```python
from build123d import *

# Parameters (mm, degrees)
F0_R      = 53.5
F0_R_2    = 10.9127793542
F1_DEPTH  = 100
F2_R      = 10.9127793542
F3_DEPTH  = 76
F5_R      = 23.9808815671
F5_R_2    = 10.9127793542
F6_DEPTH  = 50
F7_R      = 41.5
F7_R_2    = 23.9808815671
F7_R_3    = 10.9127793542
F8_DEPTH  = 11
F9_R      = 39
F9_R_2    = 10.9127793542
F10_DEPTH = 3
F11_R     = 41.5
F11_R_2   = 39
F11_R_3   = 10.9127793542
F12_DEPTH = 11
F13_R     = 5
F14_DEPTH = 125


# Not quite as in the source:
# - a feature names something its author has since deleted; it is built from what else it names


with BuildPart() as f1:
    # F0 (on Top) → F1 (new body)
    with BuildSketch(Plane.XY):
        Circle(F0_R)
        Circle(F0_R_2, mode=Mode.SUBTRACT)
    extrude(amount=F1_DEPTH)


with BuildPart() as f3:
    # F2 (on face) → F3 (new body)
    with BuildSketch(Plane.XY.offset(100)):
        with BuildLine():
            ThreePointArc((53.5, 0), (49.381382201, 20.5846810011), (37.6596601153, 38))
            Line((37.6596601153, 38), (-37.6596601153, 38))
            ThreePointArc((-37.6596601153, 38), (-53.5, 0), (-37.6596601153, -38))
            Line((-37.6596601153, -38), (37.6596601153, -38))
            ThreePointArc((37.6596601153, -38), (49.381382201, -20.5846810011), (53.5, 0))
        make_face()
        Circle(F2_R, mode=Mode.SUBTRACT)
    extrude(amount=-F3_DEPTH)


with BuildPart() as f1_1:
    add(f1.part)

    # F4: cut F3
    add(f3.part, mode=Mode.SUBTRACT)

    # F5 (on face) → F6 (join)
    with BuildSketch(Plane(origin=(0, 0, 0), x_dir=(1, 0, 0), z_dir=(0, 0, -1))):
        Circle(F5_R)
        Circle(F5_R_2, mode=Mode.SUBTRACT)
    extrude(amount=F6_DEPTH)

    # F7 (on face) → F8 (join)
    with BuildSketch(Plane(origin=(0, 0, -50), x_dir=(1, 0, 0), z_dir=(0, 0, -1))):
        Circle(F7_R)
        Circle(F7_R_2, mode=Mode.SUBTRACT)
        Circle(F7_R_2)
        Circle(F7_R_3, mode=Mode.SUBTRACT)
    extrude(amount=F8_DEPTH)

    # F9 (on face) → F10 (join)
    with BuildSketch(Plane(origin=(0, 0, -61), x_dir=(1, 0, 0), z_dir=(0, 0, -1))):
        Circle(F9_R)
        Circle(F9_R_2, mode=Mode.SUBTRACT)
    extrude(amount=F10_DEPTH)

    # F11 (on face) → F12 (join)
    with BuildSketch(Plane(origin=(0, 0, -64), x_dir=(1, 0, 0), z_dir=(0, 0, -1))):
        Circle(F11_R)
        Circle(F11_R_2, mode=Mode.SUBTRACT)
        Circle(F11_R_2)
        Circle(F11_R_3, mode=Mode.SUBTRACT)
    extrude(amount=F12_DEPTH)


with BuildPart() as f14:
    # F13 (on Front) → F14 (new body)
    with BuildSketch(Plane.XZ):
        with Locations((-63.11737746, -22.980183363)):
            Circle(F13_R)
    extrude(amount=F14_DEPTH)


with BuildPart() as f14_1:
    # F15: moved
    add(f14.part.moved(Location((63.12, 62.74391, 102))))


with BuildPart() as f1_2:
    add(f1_1.part)

    # F16: cut F14
    add(f14_1.part, mode=Mode.SUBTRACT)


solid = f1_2.part
```
The model under review builds one solid part; all positions refer to its coordinate system, in mm. A direction names the side the tool comes from. Give positions to 0.01 mm unless a question says otherwise; leave off trailing zeros. Write each loop counter-clockwise with the first axis right and the second up, starting at its lowest first coordinate (ties: lowest second). Pieces come first, ordered by that corner, then holes. Notation, with made-up numbers: (80.25, -32.5) -> (136.25, -32.5) arc R30 ccw to (136.25, -7.5) -> close; hole circle Ø10 at (-40, 48.5). An arc over 180 degrees is marked (long way). Put each result on its own line as item: value.
(1) We need section C-C, the plane z = 38. Give the boundary of the cut face in (x, y).
Results are:
outline: (-37.66, -38) arc R53.5 ccw to (37.66, -38) -> close; (-37.66, 38) -> (37.66, 38) arc R53.5 ccw to start
(2) For pin 1 Ø12 at (x, z) = (33.5, 78) entering from +Y; pin 2 Ø10 at (x, z) = (-5.5, -21) entering from -Y; pin 3 Ø22.5 at (x, z) = (12, 79) entering from +Y, all flat-tipped, find the tip position at first contact; note any pin that passes through.
Results are:
pin 1: y = 45.89
pin 2: y = -23.98
pin 3: y = 53.47
(3) We need section A-A, the plane y = 30. Give the boundary of the cut face in (x, z).
Results are:
outline: (-44.3, 0) -> (44.3, 0) -> (44.3, 24) -> (-44.3, 24) -> close; (-28.67, -75) -> (28.67, -75) -> (28.67, -64) -> (24.92, -64) -> (24.92, -61) -> (28.67, -61) -> (28.67, -50) -> (-28.67, -50) -> (-28.67, -61) -> (-24.92, -61) -> (-24.92, -64) -> (-28.67, -64) -> close
(4) Tool access review of faces 1 (the flat face through (18, 18, -50)), 2 (the flat face through (11.1, 0.5, 24)), 3 (the cylindrical face through (39.584, -12.465, -69.423)), 4 (the cylindrical face through (-0.648, -45.642, 83.977)), 5 (the flat face through (9, 9, -75)): name each direction out of +Z, -Z, +X, -X, +Y, -Y from which nothing blocks a thin tool from reaching the whole face with its end or side.
Results are:
face 1: none
face 2: +Z, +X, -X
face 3: -Z
face 4: +Y, -Y
face 5: -Z, +X, -X, +Y, -Y
(5) We need section B-B, the plane x = -34. Give the boundary of the cut face in (y, z).
Results are:
outline: (-41.31, 0) -> (41.31, 0) -> (41.31, 100) -> (38, 100) -> (38, 24) -> (-38, 24) -> (-38, 100) -> (-41.31, 100) -> close; (-23.8, -75) -> (23.8, -75) -> (23.8, -64) -> (19.1, -64) -> (19.1, -61) -> (23.8, -61) -> (23.8, -50) -> (-23.8, -50) -> (-23.8, -61) -> (-19.1, -61) -> (-19.1, -64) -> (-23.8, -64) -> close
(6) The part is to be moulded in two halves that separate along Y. For faces 6 (the cylindrical face through (39.584, -12.465, -55.423)), 7 (the cylindrical face through (-2.366, 10.653, -24.807)), 8 (the flat face through (-1, 44, 100)), say which applies: pulls with the +Y half, pulls with the -Y half, needs draft (parallel to the pull), parting line crosses it, or undercut.
Results are:
face 6: parting line crosses it
face 7: undercut
face 8: needs draft
(7) We need section D-D, the plane x = 0. State how many separate pieces and enclosed holes the cut face has, and give its area (3 significant figures).
Results are:
separate pieces: 4
enclosed holes: 0
area: 6,910 mm²
(8) To check wall thickness, follow probe 1 along X at (y, z) = (0, -54); probe 2 along X at (y, z) = (0, -31.5); probe 3 along Z at (x, y) = (14, 36). State the ranges of each line that lie inside material, in increasing order. Write a range as from..to.
Results are:
probe 1: -41.5..-10.91, 10.91..41.5
probe 2: -23.98..-10.91, 10.91..23.98
probe 3: -75..-50, 0..24
